```python
from build123d import *

# Parameters (mm, degrees)
SKETCH1_W           = 66
SKETCH1_H           = 16
SKETCH1_R           = 1.5
BOSS_EXTRUDE1_DEPTH = 1.5
SKETCH4_W           = 2.7
SKETCH4_H           = 3.35
BOSS_EXTRUDE4_DEPTH = 1.6


with BuildPart() as part:
    # Sketch1 → Boss-Extrude1 (new body)
    with BuildSketch(Plane(origin=(0, 0, 0), x_dir=(1, 0, 0), z_dir=(0, 1, 0))):
        Rectangle(SKETCH1_W, SKETCH1_H)
        with Locations((-18, -4.5)):
            Circle(SKETCH1_R, mode=Mode.SUBTRACT)
        with Locations((18, -4.5)):
            Circle(SKETCH1_R, mode=Mode.SUBTRACT)
    extrude(amount=-BOSS_EXTRUDE1_DEPTH)

    # Sketch4 → Boss-Extrude4 (add)
    with BuildSketch(Plane(origin=(0, 0, 0), x_dir=(1, 0, 0), z_dir=(0, 1, 0))):
        with Locations((-4.1, 5.425)):
            Rectangle(SKETCH4_W, SKETCH4_H)
        with Locations((4.1, 5.425)):
            Rectangle(SKETCH4_W, SKETCH4_H)
        with Locations((12.3, 5.425)):
            Rectangle(SKETCH4_W, SKETCH4_H)
        with Locations((20.5, 5.425)):
            Rectangle(SKETCH4_W, SKETCH4_H)
        with Locations((28.7, 5.425)):
            Rectangle(SKETCH4_W, SKETCH4_H)
        with Locations((-12.3, 5.425)):
            Rectangle(SKETCH4_W, SKETCH4_H)
        with Locations((-28.7, 5.425)):
            Rectangle(SKETCH4_W, SKETCH4_H)
        with Locations((-20.5, 5.425)):
            Rectangle(SKETCH4_W, SKETCH4_H)
    extrude(amount=BOSS_EXTRUDE4_DEPTH)


solid = part.part
```
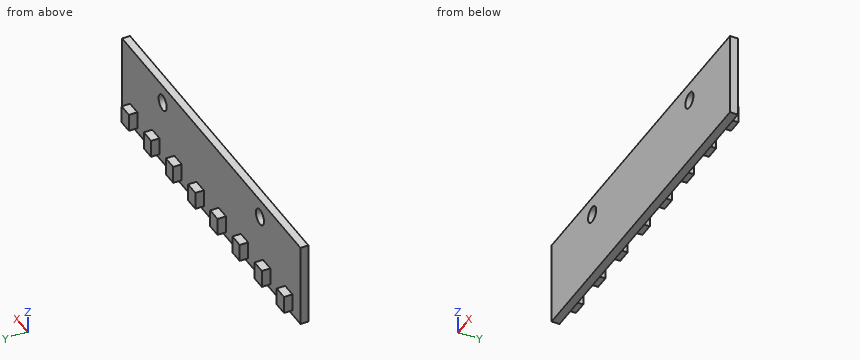
Build history of the part. All positions in model axes, mm. Round coordinates to 2 decimals unless told otherwise and drop trailing zeros. Order: outer loops, then holes, each group sorted by start corner. A loop starts at its lowest first (then second) coordinate and runs counter-clockwise, first axis right, second up. Notation, with made-up numbers: (19.25, 25) -> (34.25, 25) arc R17 ccw to (34.25, 31) -> close; hole circle Ø8 at (51, 40). An arc over 180 degrees is marked (long way). Answer in a Markdown table with one row per item.
1) Band-saw the part on D-D on x = -13. Give the cut face in (y, z).
Values:
| item | result |
|---|---|
| outline | (-1.5, -8) -> (0, -8) -> (0, -7.1) -> (1.6, -7.1) -> (1.6, -3.75) -> (0, -3.75) -> (0, 8) -> (-1.5, 8) -> close |
2) Wall check: L1, parallel to X at y = -0.4, z = 4.5; L2, parallel to Z at x = 18, y = -0.9; L3, parallel to Y at x = 24.5, z = 5.25. Give the ranges that are in metal, low to high.
Values:
| item | result |
|---|---|
| L1 | -33 to -19.5, -16.5 to 16.5, 19.5 to 33 |
| L2 | -8 to 3, 6 to 8 |
| L3 | -1.5 to 0 |
3) Pin check, flat tips, straight feed: P1, Ø0.8, axis at x = -12.5, y = 0.5, coming from the -Z side; P2, Ø1.3, axis at y = 1, z = -5, coming from the -X side; P3, Ø1.8, axis at y = 1, z = -5.5, coming from the +X side. Stop position of each tip, or through.
Values:
| item | result |
|---|---|
| P1 | z = -7.1 |
| P2 | x = -30.05 |
| P3 | x = 30.05 |
4) Band-saw the part on A-A on z = 4.5. Give the cut face in (x, y).
Values:
| item | result |
|---|---|
| outline | (-33, -1.5) -> (-19.5, -1.5) -> (-19.5, 0) -> (-33, 0) -> close; (-16.5, -1.5) -> (16.5, -1.5) -> (16.5, 0) -> (-16.5, 0) -> close; (19.5, -1.5) -> (33, -1.5) -> (33, 0) -> (19.5, 0) -> close |
5) Band-saw the part on B-B on x = 18. Give the cut face in (y, z).
Values:
| item | result |
|---|---|
| outline | (-1.5, -8) -> (0, -8) -> (0, 3) -> (-1.5, 3) -> close; (-1.5, 6) -> (0, 6) -> (0, 8) -> (-1.5, 8) -> close |
6) Band-saw the part on C-C on y = 0.75. Give the number of separate pieces and of enclosed holes in the cut face, and give its area (3 significant figures).
Values:
| item | result |
|---|---|
| separate pieces | 8 |
| enclosed holes | 0 |
| area | 72.4 mm2 |
